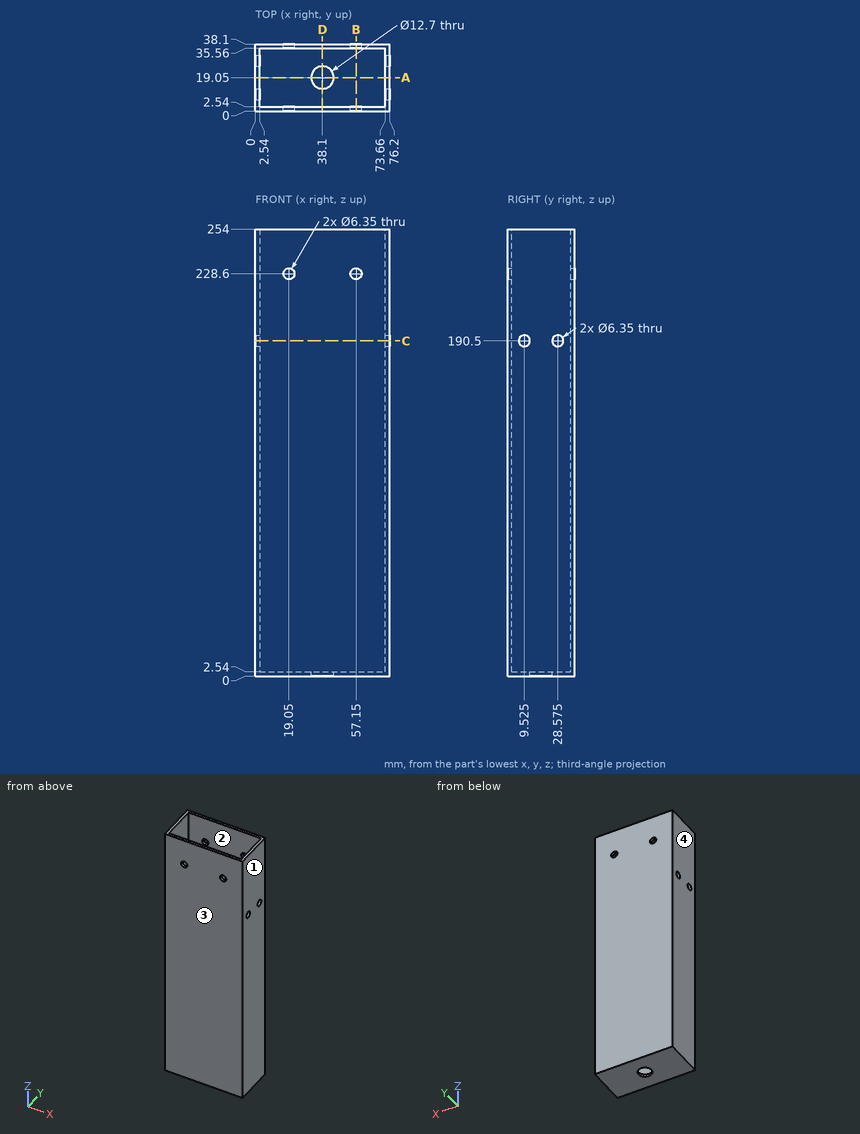
Input: dimensioned drawing with shaded views. Units: mm. Origin: part minimum x, y, z. Round coordinates to 2 decimals unless told otherwise and drop trailing zeros. Order: outer loops, then holes, each group sorted by start corner. A loop starts at its lowest first (then second) coordinate and runs counter-clockwise, first axis right, second up. Notation, with made-up numbers: (72, -11.5) - (127, -11.5) arc R25 ccw to (127, 18.5) - close; hole circle Ø5 at (31, 58). An arc over 180 degrees is marked (long way). Write item = value, one per line. Start each with the question number.
Q1. Pin query (flat end, axial travel): pin 1 (5 mm diameter, centred on x = 40.5, y = 5.5, fed in from +Z); pin 2 (4 mm diameter, centred on x = 19.05, z = 228.6, fed in from +Y). Return the tip coordinate at first contact, or that it passes through.
Q2. Ray query, line 1 (X direction, y = 36.4, z = 228.6) (3 decimals); line 2 (Y direction, x = 16, z = 68); line 3 (X direction, y = 30, z = 196). Return the intervals inside material, ascending. Write a range as from..to.
Q3. Cut plane D-D on x = 38.1. Return the cut outline in (y, z), and give its area (3 significant figures).
Q4. Cut plane A-A on y = 19.05. Return the cut outline in (x, z).
Q5. Cut plane C-C on z = 190.5. Return the cut outline in (x, y), and give its area (3 significant figures).
Q6. Cut plane B-B on x = 57.15. Return the cut outline in (y, z) (3 decimals).
Q7. Pull-direction query (X, two-part tool) for the marked faces 1, 2, 3 and 4; classes: +X half, -X half, draft (parallel to the pull), parting line (faces both ways), or undercut.
Outcome:
q1.pin_1 = 2.54
q1.pin_2 = through
q2.line_1 = 0..15.875, 22.225..53.975, 60.325..76.2
q2.line_2 = 0..2.54, 35.56..38.1
q2.line_3 = 0..2.54, 73.66..76.2
q3.outline = (0, 0) - (12.7, 0) - (12.7, 2.54) - (2.54, 2.54) - (2.54, 254) - (0, 254) - close; (25.4, 0) - (38.1, 0) - (38.1, 254) - (35.56, 254) - (35.56, 2.54) - (25.4, 2.54) - close
q3.area = 1,340 mm^2
q4.outline = (0, 0) - (31.75, 0) - (31.75, 2.54) - (2.54, 2.54) - (2.54, 254) - (0, 254) - close; (44.45, 0) - (76.2, 0) - (76.2, 254) - (73.66, 254) - (73.66, 2.54) - (44.45, 2.54) - close
q5.outline = (0, 0) - (76.2, 0) - (76.2, 6.35) - (73.66, 6.35) - (73.66, 2.54) - (2.54, 2.54) - (2.54, 6.35) - (0, 6.35) - close; (0, 12.7) - (2.54, 12.7) - (2.54, 25.4) - (0, 25.4) - close; (0, 31.75) - (2.54, 31.75) - (2.54, 35.56) - (73.66, 35.56) - (73.66, 31.75) - (76.2, 31.75) - (76.2, 38.1) - (0, 38.1) - close; (73.66, 12.7) - (76.2, 12.7) - (76.2, 25.4) - (73.66, 25.4) - close
q5.area = 490 mm^2
q6.outline = (0, 0) - (38.1, 0) - (38.1, 225.425) - (35.56, 225.425) - (35.56, 2.54) - (2.54, 2.54) - (2.54, 225.425) - (0, 225.425) - close; (0, 231.775) - (2.54, 231.775) - (2.54, 254) - (0, 254) - close; (35.56, 231.775) - (38.1, 231.775) - (38.1, 254) - (35.56, 254) - close
q7.face_1 = +X half
q7.face_2 = undercut
q7.face_3 = draft
q7.face_4 = -X half
